Work out the finished part from the listing and answer in its coordinate system (mm). Give positions to 0.01 mm unless a question says otherwise; leave off trailing zeros. Write each loop counter-clockwise with the first axis right and the second up, starting at its lowest first coordinate (ties: lowest second). Pieces come first, ordered by that corner, then holes.
1) Straight lines are drawn through the part: probe 1 along Y at (x, z) = (-25, 1.75); probe 2 along Y at (x, z) = (-15.5, 8.5); probe 3 along X at (y, z) = (-168, 4). For each, find the intervals that lie inside material, in ascending order.
2) Find section A-A (x = -104). Determine the outline of the cut face in (y, z).
3) Given pin 1 Ø1 at (y, z) = (80.5, 9) entering from -X; pin 2 Ø1.5 at (x, z) = (-204, 4.5) entering from +Y; pin 3 Ø1.5 at (y, z) = (-202.5, 3.5) entering from +X; pin 4 Ø8 at (x, y) = (1, 132) entering from -Z, each flat-ended and moving along its own axis, determine where each tip first touches the part or whether it passes through.
4) Find section B-B (y = -171.5). Determine the outline of the cut face in (x, z), plus the area to 3 significant figures.
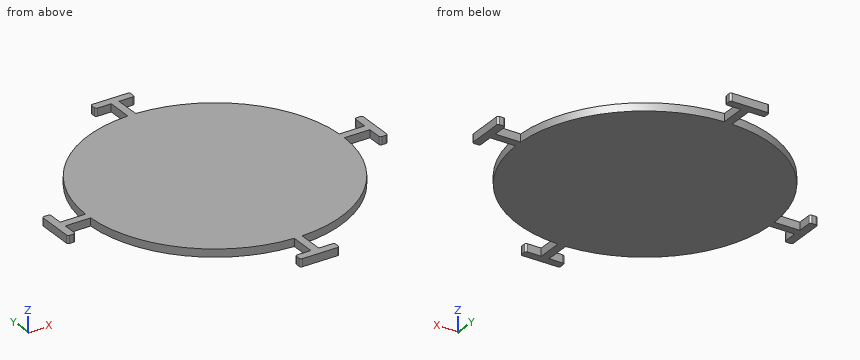
```python
from build123d import *

# Parameters (mm, degrees)
F1_DEPTH = 10.16


with BuildPart() as f1:
    # F0 (on Top) → F1 (new body)
    with BuildSketch(Plane.XY):
        with BuildLine():
            ThreePointArc((165.0218276471, -5.08), (165.080455755, -2.5403007163), (165.1, 0))
            ThreePointArc((165.1, 0), (165.080455755, 2.5403007163), (165.0218276471, 5.08))
            ThreePointArc((165.0218276471, 5.08), (116.7433295739, 116.7433295739), (5.08, 165.0218276471))
            ThreePointArc((5.08, 165.0218276471), (2.5403007163, 165.080455755), (0, 165.1))
            ThreePointArc((0, 165.1), (-2.5403007163, 165.080455755), (-5.08, 165.0218276471))
            ThreePointArc((-5.08, 165.0218276471), (-116.7433295739, 116.7433295739), (-165.0218276471, 5.08))
            ThreePointArc((-165.0218276471, 5.08), (-165.1, 0), (-165.0218276471, -5.08))
            ThreePointArc((-165.0218276471, -5.08), (-116.7433295739, -116.7433295739), (-5.08, -165.0218276471))
            ThreePointArc((-5.08, -165.0218276471), (0, -165.1), (5.08, -165.0218276471))
            ThreePointArc((5.08, -165.0218276471), (116.7433295739, -116.7433295739), (165.0218276471, -5.08))
        make_face()
        with BuildLine():
            ThreePointArc((165.0218276471, 5.08), (165.080455755, 2.5403007163), (165.1, 0))
            ThreePointArc((165.1, 0), (165.080455755, -2.5403007163), (165.0218276471, -5.08))
            Line((165.0218276471, -5.08), (198.0418276471, -5.08))
            Line((198.0418276471, -5.08), (198.0418276471, 5.08))
            Line((198.0418276471, 5.08), (165.0218276471, 5.08))
        make_face()
        with BuildLine():
            ThreePointArc((0, 165.1), (2.5403007163, 165.080455755), (5.08, 165.0218276471))
            Line((5.08, 165.0218276471), (5.08, 198.0418276471))
            Line((5.08, 198.0418276471), (-5.08, 198.0418276471))
            Line((-5.08, 198.0418276471), (-5.08, 165.0218276471))
            ThreePointArc((-5.08, 165.0218276471), (-2.5403007163, 165.080455755), (0, 165.1))
        make_face()
        with BuildLine():
            Line((198.0418276471, 22.86), (198.0418276471, 5.08))
            Line((198.0418276471, 5.08), (203.1218276471, 5.08))
            ThreePointArc((203.1218276471, 5.08), (206.713930094, 3.59210245), (208.2018276471, 4.5e-09))
            Line((208.2018276471, 4.5e-09), (208.2018276471, 22.86))
            ThreePointArc((208.2018276471, 22.86), (207.4578788713, 24.6560512242), (205.6618276471, 25.4))
            Line((205.6618276471, 25.4), (200.5818276471, 25.4))
            ThreePointArc((200.5818276471, 25.4), (198.7857764229, 24.6560512242), (198.0418276471, 22.86))
        make_face()
        with BuildLine():
            Line((203.1218276471, 5.08), (198.0418276471, 5.08))
            Line((198.0418276471, 5.08), (198.0418276471, -5.08))
            Line((198.0418276471, -5.08), (203.1218276471, -5.08))
            ThreePointArc((203.1218276471, -5.08), (206.7139300971, -3.5921024468), (208.2018276471, 4.5e-09))
            ThreePointArc((208.2018276471, 4.5e-09), (206.713930094, 3.59210245), (203.1218276471, 5.08))
        make_face()
        with BuildLine():
            Line((5.08, -198.0418276471), (5.08, -165.0218276471))
            ThreePointArc((5.08, -165.0218276471), (0, -165.1), (-5.08, -165.0218276471))
            Line((-5.08, -165.0218276471), (-5.08, -198.0418276471))
            Line((-5.08, -198.0418276471), (5.08, -198.0418276471))
        make_face()
        with BuildLine():
            Line((203.1218276471, -5.08), (198.0418276471, -5.08))
            Line((198.0418276471, -5.08), (198.0418276471, -22.86))
            ThreePointArc((198.0418276471, -22.86), (198.7857764229, -24.6560512242), (200.5818276471, -25.4))
            Line((200.5818276471, -25.4), (205.6618276471, -25.4))
            ThreePointArc((205.6618276471, -25.4), (207.4578788713, -24.6560512242), (208.2018276471, -22.86))
            Line((208.2018276471, -22.86), (208.2018276471, 4.5e-09))
            ThreePointArc((208.2018276471, 4.5e-09), (206.7139300971, -3.5921024468), (203.1218276471, -5.08))
        make_face()
        with BuildLine():
            Line((-5.08, 198.0418276471), (5.08, 198.0418276471))
            Line((5.08, 198.0418276471), (5.08, 203.1218276471))
            ThreePointArc((5.08, 203.1218276471), (3.5921024559, 206.713930088), (2.13e-08, 208.2018276471))
            ThreePointArc((2.13e-08, 208.2018276471), (-3.5921024409, 206.7139301031), (-5.08, 203.1218276471))
            Line((-5.08, 203.1218276471), (-5.08, 198.0418276471))
        make_face()
        with BuildLine():
            Line((5.08, 203.1218276471), (5.08, 198.0418276471))
            Line((5.08, 198.0418276471), (22.86, 198.0418276471))
            ThreePointArc((22.86, 198.0418276471), (24.6560512242, 198.7857764229), (25.4, 200.5818276471))
            Line((25.4, 200.5818276471), (25.4, 205.6618276471))
            ThreePointArc((25.4, 205.6618276471), (24.6560512242, 207.4578788713), (22.86, 208.2018276471))
            Line((22.86, 208.2018276471), (2.13e-08, 208.2018276471))
            ThreePointArc((2.13e-08, 208.2018276471), (3.5921024559, 206.713930088), (5.08, 203.1218276471))
        make_face()
        with BuildLine():
            Line((22.86, -198.0418276471), (5.08, -198.0418276471))
            Line((5.08, -198.0418276471), (5.08, -203.1218276471))
            ThreePointArc((5.08, -203.1218276471), (3.5921024559, -206.713930088), (2.13e-08, -208.2018276471))
            Line((2.13e-08, -208.2018276471), (22.86, -208.2018276471))
            ThreePointArc((22.86, -208.2018276471), (24.6560512242, -207.4578788713), (25.4, -205.6618276471))
            Line((25.4, -205.6618276471), (25.4, -200.5818276471))
            ThreePointArc((25.4, -200.5818276471), (24.6560512242, -198.7857764229), (22.86, -198.0418276471))
        make_face()
        with BuildLine():
            Line((5.08, -203.1218276471), (5.08, -198.0418276471))
            Line((5.08, -198.0418276471), (-5.08, -198.0418276471))
            Line((-5.08, -198.0418276471), (-5.08, -203.1218276471))
            ThreePointArc((-5.08, -203.1218276471), (-3.5921024409, -206.7139301031), (2.13e-08, -208.2018276471))
            ThreePointArc((2.13e-08, -208.2018276471), (3.5921024559, -206.713930088), (5.08, -203.1218276471))
        make_face()
        with BuildLine():
            Line((-22.86, 198.0418276471), (-5.08, 198.0418276471))
            Line((-5.08, 198.0418276471), (-5.08, 203.1218276471))
            ThreePointArc((-5.08, 203.1218276471), (-3.5921024409, 206.7139301031), (2.13e-08, 208.2018276471))
            Line((2.13e-08, 208.2018276471), (-22.86, 208.2018276471))
            ThreePointArc((-22.86, 208.2018276471), (-24.6560512242, 207.4578788713), (-25.4, 205.6618276471))
            Line((-25.4, 205.6618276471), (-25.4, 200.5818276471))
            ThreePointArc((-25.4, 200.5818276471), (-24.6560512242, 198.7857764229), (-22.86, 198.0418276471))
        make_face()
        with BuildLine():
            Line((-198.0418276471, -5.08), (-165.0218276471, -5.08))
            ThreePointArc((-165.0218276471, -5.08), (-165.1, 0), (-165.0218276471, 5.08))
            Line((-165.0218276471, 5.08), (-198.0418276471, 5.08))
            Line((-198.0418276471, 5.08), (-198.0418276471, -5.08))
        make_face()
        with BuildLine():
            Line((-5.08, -203.1218276471), (-5.08, -198.0418276471))
            Line((-5.08, -198.0418276471), (-22.86, -198.0418276471))
            ThreePointArc((-22.86, -198.0418276471), (-24.6560512242, -198.7857764229), (-25.4, -200.5818276471))
            Line((-25.4, -200.5818276471), (-25.4, -205.6618276471))
            ThreePointArc((-25.4, -205.6618276471), (-24.6560512242, -207.4578788713), (-22.86, -208.2018276471))
            Line((-22.86, -208.2018276471), (2.13e-08, -208.2018276471))
            ThreePointArc((2.13e-08, -208.2018276471), (-3.5921024409, -206.7139301031), (-5.08, -203.1218276471))
        make_face()
        with BuildLine():
            Line((-198.0418276471, -22.86), (-198.0418276471, -5.08))
            Line((-198.0418276471, -5.08), (-203.1218276471, -5.08))
            ThreePointArc((-203.1218276471, -5.08), (-206.7139300971, -3.5921024468), (-208.2018276471, 4.5e-09))
            Line((-208.2018276471, 4.5e-09), (-208.2018276471, -22.86))
            ThreePointArc((-208.2018276471, -22.86), (-207.4578788713, -24.6560512242), (-205.6618276471, -25.4))
            Line((-205.6618276471, -25.4), (-200.5818276471, -25.4))
            ThreePointArc((-200.5818276471, -25.4), (-198.7857764229, -24.6560512242), (-198.0418276471, -22.86))
        make_face()
        with BuildLine():
            Line((-203.1218276471, -5.08), (-198.0418276471, -5.08))
            Line((-198.0418276471, -5.08), (-198.0418276471, 5.08))
            Line((-198.0418276471, 5.08), (-203.1218276471, 5.08))
            ThreePointArc((-203.1218276471, 5.08), (-206.713930094, 3.59210245), (-208.2018276471, 4.5e-09))
            ThreePointArc((-208.2018276471, 4.5e-09), (-206.7139300971, -3.5921024468), (-203.1218276471, -5.08))
        make_face()
        with BuildLine():
            Line((-203.1218276471, 5.08), (-198.0418276471, 5.08))
            Line((-198.0418276471, 5.08), (-198.0418276471, 22.86))
            ThreePointArc((-198.0418276471, 22.86), (-198.7857764229, 24.6560512242), (-200.5818276471, 25.4))
            Line((-200.5818276471, 25.4), (-205.6618276471, 25.4))
            ThreePointArc((-205.6618276471, 25.4), (-207.4578788713, 24.6560512242), (-208.2018276471, 22.86))
            Line((-208.2018276471, 22.86), (-208.2018276471, 4.5e-09))
            ThreePointArc((-208.2018276471, 4.5e-09), (-206.713930094, 3.59210245), (-203.1218276471, 5.08))
        make_face()
    extrude(amount=F1_DEPTH)


solid = f1.part
```
Results:
1. probe 1: y = -207.03 to -199.21, -163.2 to 163.2, 199.21 to 207.03
1. probe 2: y = -208.2 to -198.04, -164.37 to 164.37, 198.04 to 208.2
1. probe 3: x = -5.08 to 5.08
2. outline: (-128.23, 0) - (128.23, 0) - (128.23, 10.16) - (-128.23, 10.16) - close
3. pin 1: stops at x = -144.42
3. pin 2: stops at y = 25.4
3. pin 3: stops at x = 25.4
3. pin 4: stops at z = 0
4. outline: (-5.08, 0) - (5.08, 0) - (5.08, 10.16) - (-5.08, 10.16) - close
4. area: 103 mm2
